```python
from build123d import *

# Parameters (mm, degrees)
SKETCH1_W           = 20.14
SKETCH1_H           = 23
BOSS_EXTRUDE1_DEPTH = 1.66
SKETCH2_W           = 8.04
SKETCH2_H           = 6.62
BOSS_EXTRUDE2_DEPTH = 7.55
SKETCH3_W           = 10.1
SKETCH3_H           = 7.64
BOSS_EXTRUDE3_DEPTH = 5.13
FILLET1_R           = 2
HOLE1_D             = 2.6


with BuildPart() as part:
    # Sketch1 → Boss-Extrude1 (new body)
    with BuildSketch(Plane(origin=(0, 0, 0), x_dir=(1, 0, 0), z_dir=(0, 1, 0))):
        with Locations((0, 0.178988327)):
            Rectangle(SKETCH1_W, SKETCH1_H)
    extrude(amount=BOSS_EXTRUDE1_DEPTH)

    # Sketch2 → Boss-Extrude2 (add)
    with BuildSketch(Plane.XZ):
        with Locations((0, 8.011011673)):
            Rectangle(SKETCH2_W, SKETCH2_H)
    extrude(amount=-BOSS_EXTRUDE2_DEPTH)

    # Sketch3 → Boss-Extrude3 (add)
    with BuildSketch(Plane.XZ):
        with Locations((0, -9.498988327)):
            Rectangle(SKETCH3_W, SKETCH3_H)
    extrude(amount=-BOSS_EXTRUDE3_DEPTH)

    # Fillet1
    fillet1_edges = [part.edges().sort_by_distance(p)[0] for p in [
        (-10.07, 0.83, -11.678988327),
        (10.07, 0.83, -11.678988327),
        (10.07, 0.83, 11.321011673),
        (-10.07, 0.83, 11.321011673),
    ]]
    fillet(fillet1_edges, radius=FILLET1_R)

    # Hole1 (through all)
    with Locations(Plane(origin=(0, 1.66, 0), x_dir=(1, 0, 0), z_dir=(0, 1, 0))):
        with Locations((-7.2, 8.965942289), (7.2, 8.965942289), (7.2, -8.68646887), (-7.2, -8.68646887)):
            Hole(HOLE1_D / 2)


solid = part.part
```
Input: part model. Units: mm. Frame: model coordinates. A direction names the side the tool comes from. Round coordinates to 2 decimals unless told otherwise and drop trailing zeros. Loops run counter-clockwise (first coordinate to the right, second up) from the corner with the lowest first, then second, coordinate; pieces in that order, holes last.
1) Section query C-C on x = -4.5. Return the cut outline in (y, z).
Ans:
outline: (0, -13.32) - (5.13, -13.32) - (5.13, -5.68) - (1.66, -5.68) - (1.66, 11.32) - (0, 11.32) - close
2) Section query B-B on z = 9. Return the cut outline in (x, y).
Ans:
outline: (-10.07, 0) - (-8.46, 0) - (-8.46, 1.66) - (-10.07, 1.66) - close; (-5.94, 0) - (5.94, 0) - (5.94, 1.66) - (4.02, 1.66) - (4.02, 7.55) - (-4.02, 7.55) - (-4.02, 1.66) - (-5.94, 1.66) - close; (8.46, 0) - (10.07, 0) - (10.07, 1.66) - (8.46, 1.66) - close
3) Material intervals for line 1 (Z direction, x = 7.2, y = 1.2); line 2 (Z direction, x = 3.75, y = 5); line 3 (Y direction, x = -4.5, z = 8), sorted ascending.
Ans:
line 1: z = -11.68 to -10.27, -7.67 to 7.39, 9.99 to 11.32
line 2: z = -13.32 to -5.68, 4.7 to 11.32
line 3: y = 0 to 1.66
4) Set-up query: faces 4 (the flat face through (7, 1, -11.679)), 5 (the flat face through (0, 5.13, -9)), 6 (the flat face through (-4.02, 5, 8)). Return all of +Z, -Z, +X, -X, +Y, -Y with unobstructed straight access to the full face (end or side cutting, diameter ignored); none if empty.
Ans:
face 4: -Z, +X, +Y, -Y
face 5: -Z, +X, -X, +Y
face 6: +Z, -X, +Y
5) Section query D-D on y = 5.5. Return the cut outline in (x, z), plus the area to 3 significant figures.
Ans:
outline: (-4.02, 4.7) - (4.02, 4.7) - (4.02, 11.32) - (-4.02, 11.32) - close
area: 53.2 mm2
6) Pin query (flat end, axial travel): pin 1 (1.5 mm diameter, centred on y = 3, z = -8, fed in from -X); pin 2 (1.5 mm diameter, centred on y = 3, z = -10, fed in from +X); pin 3 (4 mm diameter, centred on x = 2, z = -8, fed in from +Y). Return the tip coordinate at first contact, or that it passes through.
Ans:
pin 1: stops at x = -5.05
pin 2: stops at x = 5.05
pin 3: stops at y = 5.13
7) Section query A-A on x = 7.2. Return the cut outline in (y, z).
Ans:
outline: (0, -11.68) - (1.66, -11.68) - (1.66, -10.27) - (0, -10.27) - close; (0, -7.67) - (1.66, -7.67) - (1.66, 7.39) - (0, 7.39) - close; (0, 9.99) - (1.66, 9.99) - (1.66, 11.32) - (0, 11.32) - close
8) Pull-direction query (Z, two-part tool) for faces 1 (the cylindrical face through (-9.5, 0.84, 10.72)), 2 (the flat face through (0, 3, -5.679)), 3 (the flat face through (-7, 1, -11.679)); classes: released by +Z, released by -Z, zero draft, split by the parting line, or undercut.
Ans:
face 1: released by +Z
face 2: undercut
face 3: released by -Z
